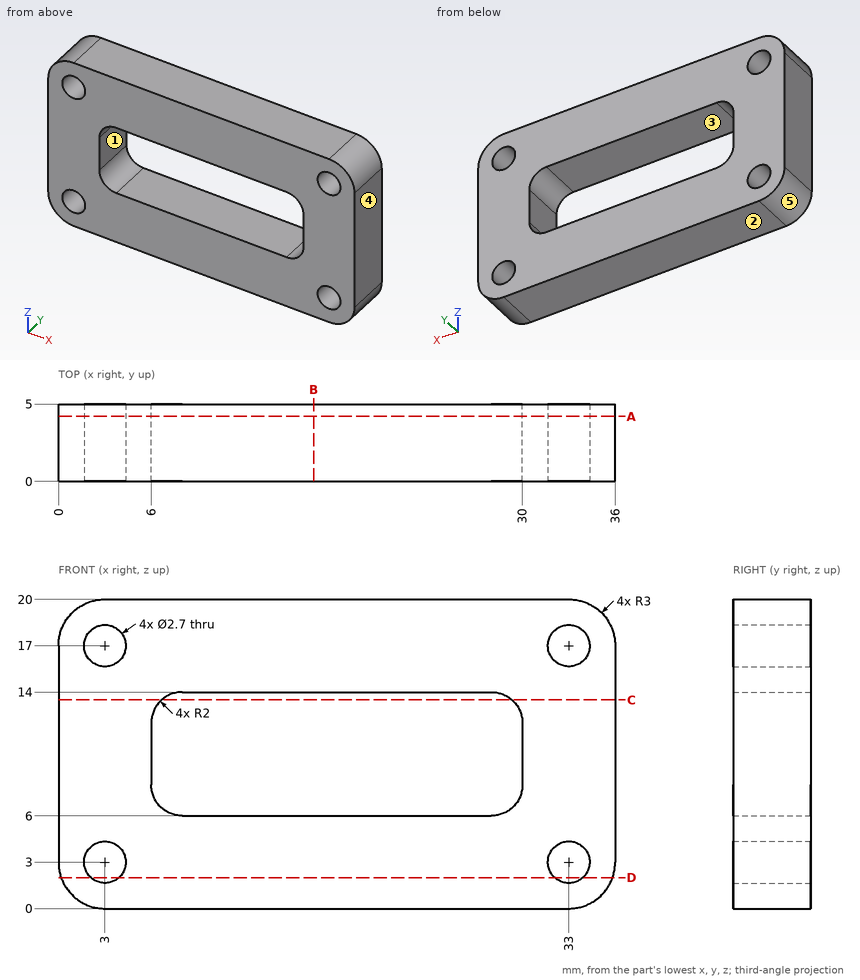
The figure shows three views and two pictorial views of one solid part (mm, origin at its lowest corner). Answer the questions. A direction names the side the tool comes from. Coordinates: 2 decimals unless noted, no trailing zeros. Loops run counter-clockwise (first coordinate to the right, second up) from the corner with the lowest first, then second, coordinate; pieces in that order, holes last.
1) Find section C-C on z = 13.5. Write down the section's boundary in (x, y).
2) Find the intervals of material crossed by L1, parallel to X at y = 1.3, z = 3; L2, parallel to Z at x = 8.5, y = 4.4; L3, parallel to Z at x = 3.5, y = 3.4, in increasing order.
3) Find section B-B on x = 16.5. Write down the section's boundary in (y, z), then the cut area to 3 significant figures.
4) Find section D-D on z = 2. Write down the section's boundary in (x, y).
5) Find section A-A on y = 4.2. Write down the section's boundary in (x, z), then the cut area to 3 significant figures.
6) A tool of negligible diameter and unlimited length cuts with its end or side. For the marked faces 1 and 2, from which of +Z, -Z, +X, -X, +Y, -Y can it reach the whole face along a straight path? Write none if from no direction.
7) A flat-ended cylindrical pin translates along its axis: pin 1 Ø2 at (x, z) = (3, 3) entering from +Y. Find the tip coordinate at first contact, or state that the pin passes through.
8) Determine the mould class of the marked faces 3, 4 and 5 for opening direction Z: pulls with the +Z half, pulls with the -Z half, needs draft (parallel to the pull), parting line crosses it, or undercut.
Values:
1. outline: (0, 0) - (6.68, 0) - (6.68, 5) - (0, 5) - close; (29.32, 0) - (36, 0) - (36, 5) - (29.32, 5) - close
2. L1: x = 0 to 1.65, 4.35 to 31.65, 34.35 to 36
2. L2: z = 0 to 6, 14 to 20
2. L3: z = 0 to 1.75, 4.25 to 15.75, 18.25 to 20
3. outline: (0, 0) - (5, 0) - (5, 6) - (0, 6) - close; (0, 14) - (5, 14) - (5, 20) - (0, 20) - close
3. area: 60.0 mm2
4. outline: (0.17, 0) - (2.09, 0) - (2.09, 5) - (0.17, 5) - close; (3.91, 0) - (32.09, 0) - (32.09, 5) - (3.91, 5) - close; (33.91, 0) - (35.83, 0) - (35.83, 5) - (33.91, 5) - close
5. outline: (0, 3) arc R3 ccw to (3, 0) - (33, 0) arc R3 ccw to (36, 3) - (36, 17) arc R3 ccw to (33, 20) - (3, 20) arc R3 ccw to (0, 17) - close; hole circle Ø2.7 at (3, 3); hole circle Ø2.7 at (3, 17); hole (6, 8) arc R2 ccw to (8, 6) - (28, 6) arc R2 ccw to (30, 8) - (30, 12) arc R2 ccw to (28, 14) - (8, 14) arc R2 ccw to (6, 12) - close; hole circle Ø2.7 at (33, 3); hole circle Ø2.7 at (33, 17)
5. area: 501 mm2
6. face 1: +Y, -Y
6. face 2: -Z, +X, -X, +Y, -Y
7. pin 1: passes through
8. face 3: undercut
8. face 4: needs draft
8. face 5: pulls with the -Z half
